```python
from build123d import *

# Parameters (mm, degrees)
BOSS_EXTRUDE3_DEPTH = 12.7
SKETCH8_R           = 2
CUT_EXTRUDE5_DEPTH  = 12.7
CUT_EXTRUDE7_DEPTH  = 12.7
SKETCH10_W          = 12.7
SKETCH10_H          = 5.08
BOSS_EXTRUDE4_DEPTH = 6.35
SKETCH11_R          = 1.5875
CUT_EXTRUDE8_DEPTH  = 12.7
SKETCH13_R          = 3
SKETCH13_R_2        = 2
BOSS_EXTRUDE5_DEPTH = 1.27
CUT_EXTRUDE10_DEPTH = 0.254


with BuildPart() as part:
    # Sketch7 → Boss-Extrude3 (new body)
    with BuildSketch(Plane.XY):
        Polygon((0, 8.571363245), (12.192, 28.082641823), (24.892, 28.082641823), (12.7, 8.571363245), (12.7, 0), (0, 0), align=None)
    extrude(amount=BOSS_EXTRUDE3_DEPTH)

    # Sketch8 → Cut-Extrude5 (cut)
    with BuildSketch(Plane(origin=(-3.851945127, 2.406962455, 0), x_dir=(0, 0, 1), z_dir=(-0.848048096, 0.529919264, 0))):
        with Locations((6.35, 18.772567442)):
            Circle(SKETCH8_R)
    extrude(amount=-CUT_EXTRUDE5_DEPTH, mode=Mode.SUBTRACT)

    # Sketch9 → Cut-Extrude7 (cut)
    with BuildSketch(Plane.XY.offset(12.7)):
        Polygon((21.717663692, 23.002641823), (9.017663692, 23.002641823), (12.192, 28.082641823), (24.892, 28.082641823), align=None)
    extrude(amount=-CUT_EXTRUDE7_DEPTH, mode=Mode.SUBTRACT)

    # Sketch10 → Boss-Extrude4 (add)
    with BuildSketch(Plane.XY.offset(12.7)):
        with Locations((6.35, 2.54)):
            Rectangle(SKETCH10_W, SKETCH10_H)
    boss_extrude4 = extrude(amount=BOSS_EXTRUDE4_DEPTH)

    # Sketch11 → Cut-Extrude8 (cut)
    with BuildSketch(Plane(origin=(0, 5.08, 0), x_dir=(1, 0, 0), z_dir=(0, 1, 0))):
        with Locations((6.35, -15.875)):
            Circle(SKETCH11_R)
    cut_extrude8 = extrude(amount=-CUT_EXTRUDE8_DEPTH, mode=Mode.SUBTRACT)

    # Mirror2: Boss-Extrude4, Cut-Extrude8 across plane
    add(boss_extrude4.mirror(Plane.XY.offset(6.35)))
    add(cut_extrude8.mirror(Plane.XY.offset(6.35)), mode=Mode.SUBTRACT)

    # Sketch13 → Boss-Extrude5 (add)
    with BuildSketch(Plane(origin=(-3.851945127, 2.406962455, 0), x_dir=(0, 0, 1), z_dir=(-0.848048096, 0.529919264, 0))):
        with Locations((6.35, 18.772567442)):
            Circle(SKETCH13_R)
        with Locations((6.35, 18.772567442)):
            Circle(SKETCH13_R_2, mode=Mode.SUBTRACT)
    extrude(amount=BOSS_EXTRUDE5_DEPTH)

    # Sketch17 → Cut-Extrude10 (cut)
    with BuildSketch(Plane(origin=(0, 23.002641823, 0), x_dir=(1, 0, 0), z_dir=(0, 1, 0))):
        with BuildLine():
            Line((14.380484205, -6.35), (14.380484205, -2.85))
            Line((14.380484205, -2.85), (14.941381641, -2.85))
            add(Edge.make_bspline(
                [(14.941381641, -2.85), (14.980647969, -2.849995519), (15.056627568, -2.849986848), (15.166246302, -2.853836298), (15.267908419, -2.858815992), (15.361290393, -2.864387113), (15.446551165, -2.873987267), (15.523561083, -2.88410478), (15.592474012, -2.896305878), (15.635079132, -2.907250641), (15.655123628, -2.91239984)],
                knots=[0, 0, 0, 0, 0.000117791, 0.000227922, 0.000329003, 0.000423165, 0.000508489, 0.000586326, 0.000656186, 0.000718254, 0.000718254, 0.000718254, 0.000718254], degree=3))
            add(Edge.make_bspline(
                [(15.655123628, -2.91239984), (15.681444087, -2.919662877), (15.733093276, -2.933915288), (15.807071397, -2.962698647), (15.877249964, -2.994693392), (15.943543291, -3.031193412), (16.005544311, -3.072639364), (16.063017398, -3.119360176), (16.117202106, -3.169480477), (16.166174458, -3.224397106), (16.210437395, -3.282426696), (16.248893952, -3.343554044), (16.28230777, -3.406844471), (16.309047578, -3.473094446), (16.32919552, -3.54199887), (16.343931641, -3.61326351), (16.353482643, -3.687113865), (16.354385087, -3.737356675), (16.354843179, -3.762860577)],
                knots=[0, 0, 0, 0, 8.1863e-05, 0.000160642, 0.000237816, 0.000313134, 0.000387417, 0.000461218, 0.000535129, 0.000608609, 0.000681668, 0.000753832, 0.000825019, 0.000896106, 0.000967761, 0.001040089, 0.001114269, 0.001190743, 0.001190743, 0.001190743, 0.001190743], degree=3))
            add(Edge.make_bspline(
                [(16.354843179, -3.762860577), (16.353645404, -3.795626396), (16.351287729, -3.860121885), (16.336226745, -3.954854089), (16.307985053, -4.044389639), (16.271031486, -4.130378639), (16.220786188, -4.212500352), (16.156984378, -4.290715729), (16.080659434, -4.367433141), (16.022113989, -4.413420054), (15.99166209, -4.437339744)],
                knots=[0, 0, 0, 0, 9.8317e-05, 0.000193525, 0.000286672, 0.000379289, 0.00047368, 0.000574417, 0.000681503, 0.000797579, 0.000797579, 0.000797579, 0.000797579], degree=3))
            add(Edge.make_bspline(
                [(15.99166209, -4.437339744), (16.016338848, -4.449937015), (16.064723145, -4.474636779), (16.133414631, -4.515235817), (16.197015449, -4.558418043), (16.255810766, -4.603314613), (16.308567282, -4.651828759), (16.357463403, -4.701165027), (16.400086847, -4.754150182), (16.438202016, -4.808895731), (16.471331101, -4.866194396), (16.500182881, -4.925949414), (16.524552945, -4.988364919), (16.545190145, -5.053123267), (16.560581374, -5.120447198), (16.570616783, -5.190360788), (16.57830052, -5.262625597), (16.578898242, -5.311850581), (16.579202154, -5.336879006)],
                knots=[0, 0, 0, 0, 8.3106e-05, 0.000162948, 0.000239177, 0.000313644, 0.000384624, 0.000454039, 0.000521819, 0.000588334, 0.000653992, 0.000720158, 0.00078721, 0.000854842, 0.000923894, 0.000994098, 0.001066653, 0.001141702, 0.001141702, 0.001141702, 0.001141702], degree=3))
            add(Edge.make_bspline(
                [(16.579202154, -5.336879006), (16.577229969, -5.384681869), (16.573337872, -5.479020625), (16.544880751, -5.617531587), (16.495545146, -5.748852541), (16.429297601, -5.872461563), (16.34766788, -5.984780374), (16.25381711, -6.083170677), (16.148690152, -6.166455884), (16.051697827, -6.222666938), (15.967807104, -6.260389811), (15.898321986, -6.28371247), (15.823696442, -6.305318547), (15.742563511, -6.32049078), (15.656394023, -6.334378075), (15.564347819, -6.34295238), (15.466596934, -6.348762974), (15.3994574, -6.349579322), (15.364859205, -6.35)],
                knots=[0, 0, 0, 0, 0.000143365, 0.000282931, 0.000422024, 0.000562867, 0.000702406, 0.000837288, 0.000969562, 0.001103403, 0.001172455, 0.001245183, 0.001323096, 0.001405322, 0.001492583, 0.001584881, 0.001682498, 0.001786285, 0.001786285, 0.001786285, 0.001786285], degree=3))
            Line((15.364859205, -6.35), (14.380484205, -6.35))
        make_face()
        with BuildLine():
            Line((15.008689333, -3.478205128), (15.008689333, -4.241025641))
            Line((15.008689333, -4.241025641), (15.175556321, -4.241025641))
            add(Edge.make_bspline(
                [(15.175556321, -4.241025641), (15.198235043, -4.240827874), (15.242014945, -4.240446097), (15.305250369, -4.235528937), (15.364049102, -4.227139958), (15.418188132, -4.215435223), (15.468171784, -4.200571914), (15.513680747, -4.182688154), (15.554514928, -4.160868022), (15.601954802, -4.128365973), (15.65210217, -4.080537752), (15.696246334, -4.011439977), (15.722246952, -3.9319778), (15.725142719, -3.875934919), (15.726638051, -3.846995192)],
                knots=[0, 0, 0, 0, 6.8023e-05, 0.000131315, 0.000190113, 0.000246084, 0.000297324, 0.000346407, 0.000392516, 0.000435884, 0.000518691, 0.000598437, 0.000679585, 0.000766233, 0.000766233, 0.000766233, 0.000766233], degree=3))
            add(Edge.make_bspline(
                [(15.726638051, -3.846995192), (15.725441512, -3.81988833), (15.723128051, -3.7674783), (15.696948772, -3.693889951), (15.656287176, -3.628675613), (15.608280446, -3.584041731), (15.563072782, -3.553558106), (15.524363206, -3.533485938), (15.481876539, -3.515517537), (15.434790286, -3.50177846), (15.383373334, -3.491469141), (15.327875445, -3.48389818), (15.268200865, -3.478745062), (15.226983506, -3.478388967), (15.205704558, -3.478205128)],
                knots=[0, 0, 0, 0, 8.0997e-05, 0.000156604, 0.000231296, 0.000309653, 0.000351072, 0.000394666, 0.000440239, 0.000489262, 0.000541514, 0.000597437, 0.000657234, 0.000721051, 0.000721051, 0.000721051, 0.000721051], degree=3))
            Line((15.205704558, -3.478205128), (15.008689333, -3.478205128))
        make_face(mode=Mode.SUBTRACT)
        with BuildLine():
            Line((15.008689333, -4.824358974), (15.008689333, -5.721794872))
            Line((15.008689333, -5.721794872), (15.189578756, -5.721794872))
            add(Edge.make_bspline(
                [(15.189578756, -5.721794872), (15.225340826, -5.721590564), (15.294097866, -5.721197758), (15.392592205, -5.716451722), (15.482148183, -5.707897829), (15.56252851, -5.697218983), (15.633856304, -5.682750816), (15.695890459, -5.664356397), (15.749481695, -5.644119331), (15.794308675, -5.619124153), (15.830929749, -5.590035963), (15.863976429, -5.560307135), (15.890920633, -5.526012123), (15.91223939, -5.488623117), (15.930690736, -5.449068886), (15.941819286, -5.405804853), (15.950292172, -5.36011326), (15.950758458, -5.328509373), (15.950997026, -5.312339744)],
                knots=[0, 0, 0, 0, 0.000107281, 0.000206261, 0.0002957, 0.000377105, 0.000449433, 0.000513769, 0.000571055, 0.000620973, 0.00066697, 0.000711118, 0.000754041, 0.00079709, 0.000840088, 0.000884486, 0.000930707, 0.00097913, 0.00097913, 0.00097913, 0.00097913], degree=3))
            add(Edge.make_bspline(
                [(15.950997026, -5.312339744), (15.950470915, -5.293849518), (15.949446194, -5.257835532), (15.941077284, -5.205197249), (15.925868241, -5.156055919), (15.906711709, -5.109154932), (15.880054377, -5.066173507), (15.848373048, -5.02562422), (15.810093916, -4.988880195), (15.767046798, -4.953719015), (15.716836597, -4.922933498), (15.659439756, -4.896221608), (15.594544464, -4.873912821), (15.5219497, -4.856150551), (15.441973715, -4.841075958), (15.354032772, -4.832074761), (15.258859273, -4.825380176), (15.19286442, -4.82470711), (15.158729397, -4.824358974)],
                knots=[0, 0, 0, 0, 5.546e-05, 0.00010802, 0.00015926, 0.000209526, 0.000259547, 0.000310464, 0.000363513, 0.000418371, 0.000476935, 0.000539665, 0.000607959, 0.000682439, 0.000763712, 0.0008519, 0.000947461, 0.001049847, 0.001049847, 0.001049847, 0.001049847], degree=3))
            Line((15.158729397, -4.824358974), (15.008689333, -4.824358974))
        make_face(mode=Mode.SUBTRACT)
    extrude(amount=-CUT_EXTRUDE10_DEPTH, mode=Mode.SUBTRACT)


solid = part.part
```
Geometry check sheet. Reference: the model listing, model coordinates, mm. A direction names the side the tool comes from. Coordinates: 2 decimals unless noted, no trailing zeros. Loops run counter-clockwise (first coordinate to the right, second up) from the corner with the lowest first, then second, coordinate; pieces in that order, holes last.
Item 1: Thickness scan on line 1 (Z direction, x = 6.35, y = 1.6); line 2 (X direction, y = 3.5, z = -1.25); line 3 (Y direction, x = 1, z = 15.75). Record the ranges inside material, lowest first.
Item 2: Sectioned sample at B-B, the plane y = 3. Count the separate pieces of the cut face and the enclosed holes in it, then the cut area to 3 significant figures.
Item 3: Access from +Z, -Z, +X, -X, +Y, -Y to the whole of each face (thin tool, end or side, straight path). Record for faces 5 (the face through (6, 0, 7)), 6 (the face through (12.7, 3, 7)), 7 (the face through (5, 5.08, -2)), 8 (the face through (5, 5.08, 17)), 9 (the face through (6.006, 2.576, 17.425)).
Item 4: Go/stop test with flat-tipped pins: pin 1 Ø3 at (x, z) = (7.5, -2.5) entering from +Y; pin 2 Ø8 at (x, z) = (2.5, 8) entering from +Y; pin 3 Ø4 at (y, z) = (10, 14.5) entering from +X; pin 4 Ø1 at (x, y) = (16.5, 12.5) entering from +Z. Record where each tip stops, or that it passes through.
Item 5: Sectioned sample at D-D, the plane y = 10.25. Record the boundary of the cut face in (x, z).
Item 6: Release check for a two-part mould opening along Z. For faces 1 (the face through (15.3, 22.749, 4.6)), 2 (the face through (6, 3, -6.35)), 3 (the face through (0, 3, 7)), 4 (the face through (6.906, 20.804, 7.963)) record: released by +Z, released by -Z, zero draft, split by the parting line, or undercut.
Item 7: Sectioned sample at A-A, the plane z = 7.5. Record the boundary of the cut face in (x, y), then the cut area to 3 significant figures.
Item 8: Sectioned sample at C-C, the plane z = 16.5. Record the boundary of the cut face in (x, y).
Check result:
1. line 1: z = -6.35 to -4.76, -1.59 to 14.29, 17.46 to 19.05
1. line 2: x = 0 to 12.7
1. line 3: y = 0 to 5.08
2. separate pieces: 1
2. enclosed holes: 2
2. area: 307 mm2
3. face 5: +Z, -Z, +X, -X, -Y
3. face 6: +Z, -Z, +X, -Y
3. face 7: -Z, +X, -X, +Y
3. face 8: +Z, +X, -X, +Y
3. face 9: +Y, -Y
4. pin 1: stops at y = 5.08
4. pin 2: stops at y = 21.33
4. pin 3: stops at x = 14.14
4. pin 4: passes through
5. outline: (1.05, 0) - (13.75, 0) - (13.75, 12.7) - (1.05, 12.7) - close
6. face 1: undercut
6. face 2: released by -Z
6. face 3: zero draft
6. face 4: split by the parting line
7. outline: (0, 0) - (12.7, 0) - (12.7, 8.57) - (14.36, 11.23) - (4.15, 17.61) - (3.55, 16.65) - (4.63, 15.98) - (0, 8.57) - close; (5.89, 20.39) - (16.1, 14.01) - (21.72, 23) - (9.02, 23) - (7.56, 20.68) - (6.49, 21.35) - close
7. area: 260 mm2
8. outline: (0, 0) - (4.89, 0) - (4.89, 5.08) - (0, 5.08) - close; (7.81, 0) - (12.7, 0) - (12.7, 5.08) - (7.81, 5.08) - close
